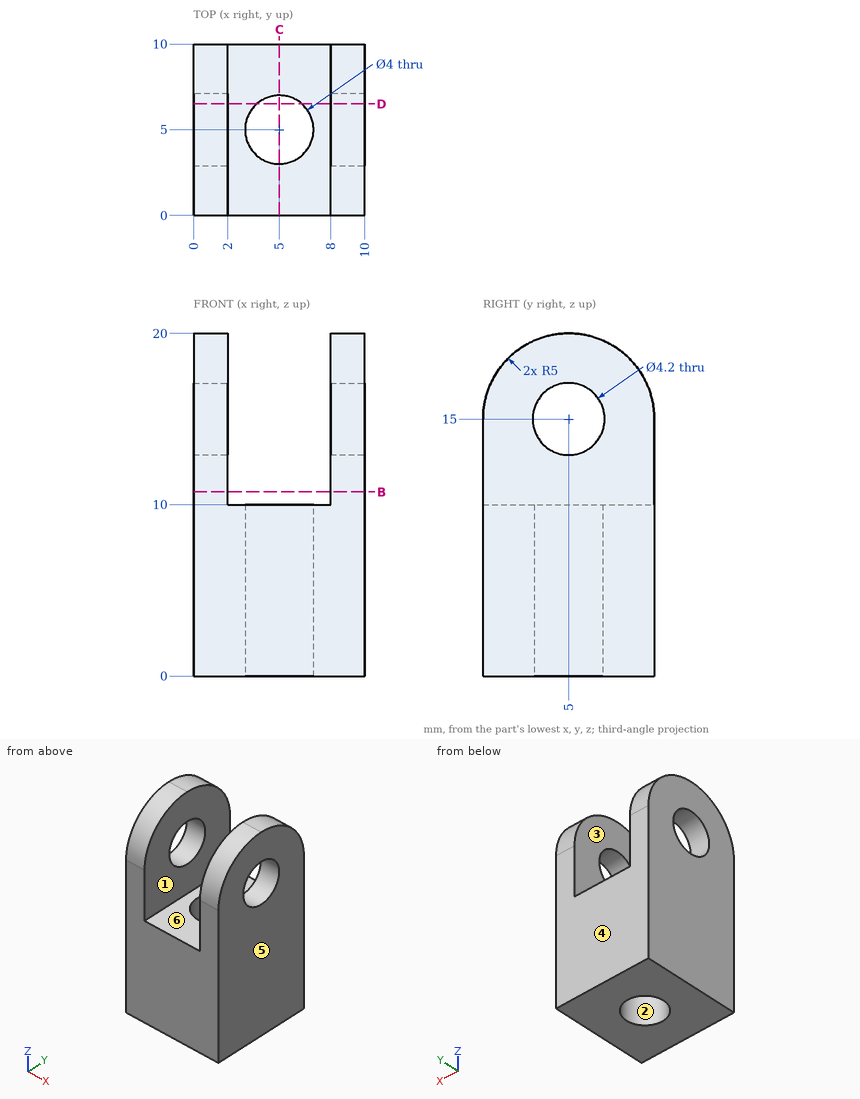
Geometry check sheet. Reference: drawing and pictorial views, mm from the part's lowest x, y, z. A direction names the side the tool comes from. Round coordinates to 2 decimals unless told otherwise and drop trailing zeros. Order: outer loops, then holes, each group sorted by start corner. A loop starts at its lowest first (then second) coordinate and runs counter-clockwise, first axis right, second up. Notation, with made-up numbers: (-38, 62.5) - (-8, 62.5) arc R9 cw to (-8, 69.5) - close; hole circle Ø3 at (26, 70.25). An arc over 180 degrees is marked (long way). Write item = value, one per line.
Q1. Section check B-B (z = 10.75). Record the boundary of the cut face in (x, y).
Computed:
outline = (0, 0) - (2, 0) - (2, 10) - (0, 10) - close; (8, 0) - (10, 0) - (10, 10) - (8, 10) - close
Q2. Section check D-D (y = 6.5). Record the boundary of the cut face in (x, z), and give its area (3 significant figures).
Computed:
outline = (0, 0) - (3.68, 0) - (3.68, 10) - (2, 10) - (2, 13.53) - (0, 13.53) - close; (0, 16.47) - (2, 16.47) - (2, 19.77) - (0, 19.77) - close; (6.32, 0) - (10, 0) - (10, 13.53) - (8, 13.53) - (8, 10) - (6.32, 10) - close; (8, 16.47) - (10, 16.47) - (10, 19.77) - (8, 19.77) - close
area = 101 mm^2
Q3. Thickness scan on line 1 along Y through (x, z) = (5, 6.5); line 2 along X through (y, z) = (1.75, 13.75); line 3 along Z through (x, y) = (0.8, 5). Record the ranges inside material, lowest first.
Computed:
line_1 = 0 to 3, 7 to 10
line_2 = 0 to 2, 8 to 10
line_3 = 0 to 12.9, 17.1 to 20
Q4. Section check C-C (x = 5). Record the boundary of the cut face in (y, z).
Computed:
outline = (0, 0) - (3, 0) - (3, 10) - (0, 10) - close; (7, 0) - (10, 0) - (10, 10) - (7, 10) - close
Q5. Go/stop test with flat-tipped pins: pin 1 (5 mm diameter, centred on x = 8.5, y = 5, fed in from -Z); pin 2 (3 mm diameter, centred on x = 6, y = 5, fed in from +Z). Record where each tip stops, or that it passes through.
Computed:
pin_1 = 0
pin_2 = 10
Q6. Tool access check on the marked faces 1 and 2. Record the directions out of +Z, -Z, +X, -X, +Y, -Y that give a thin tool (end or side, any length) a straight path to the whole face; none if there is none.
Computed:
face_1 = +Z, +Y, -Y
face_2 = +Z, -Z
Q7. Draft check along X on the marked faces 3, 4, 5 and 6. Enter one of: pulls with the +X half, pulls with the -X half, needs draft (parallel to the pull), parting line crosses it, or undercut.
Computed:
face_3 = undercut
face_4 = needs draft
face_5 = pulls with the +X half
face_6 = undercut
